Here's how the part is built. I have some questions about the finished solid (model axes, mm). A direction names the side the tool comes from. Give positions to 0.01 mm unless a question says otherwise; leave off trailing zeros. Loops run counter-clockwise (first coordinate to the right, second up) from the corner with the lowest first, then second, coordinate; pieces in that order, holes last.
Q1. I'm going to push flat-ended pins straight in: P1, Ø7.5, axis at x = -4.5, z = -5, coming from the +Y side; P2, Ø4, axis at x = 7.5, y = -52.5, coming from the +Z side (3 decimals); P3, Ø1, axis at x = 1.5, z = 5, coming from the +Y side. Where does each tip first touch, or does it pass through?
Q2. Suppose I cut it at A-A (z = 0). List the corners of the cut face in (x, y) for me, and give its area (3 significant figures).
Q3. Suppose I cut it at C-C (y = -17). List the corners of the cut face in (x, z) for me, and give its area (3 significant figures).
Q4. Thinking about a two-plate mould opening in Y: for faces 1 (the face through (0, -60, 0)), 2 (the face through (-2, 8, 0)), 3 (the face through (0, 12.3, 0)), which applies, pulls with the +Y half, pulls with the -Y half, needs draft (parallel to the pull), parting line crosses it, or undercut?
Q5. For faces 4 (the face through (3.755, -29.58, 11.923)), 5 (the face through (-3.417, 1.479, -0.759)), which set-ups out of +Z, -Z, +X, -X, +Y, -Y let a thin tool reach every point of the face, with its end or its side?
Q6. I need wall thicknesses on probe 1 along Y at (x, z) = (5.5, -2); probe 2 along X at (y, z) = (-38, 0); probe 3 along Z at (x, y) = (9, -40). Which ranges of each line are inside material? Lowest first, please.
Q7. Suppose I cut it at D-D (z = -7.5). List the corners of the cut face in (x, y) for me.
Q8. Suppose I cut it at B-B (x = 0). List the corners of the cut face in (y, z) for me.
```python
from build123d import *

# Parameters (mm, degrees)
SKETCH1_R           = 12.5
BOSS_EXTRUDE1_DEPTH = 60
SKETCH2_R           = 3.5
BOSS_EXTRUDE2_DEPTH = 3
SKETCH3_R           = 2
BOSS_EXTRUDE3_DEPTH = 9.3


with BuildPart() as part:
    # Sketch1 → Boss-Extrude1 (new body)
    with BuildSketch(Plane(origin=(0, 0, 0), x_dir=(1, 0, 0), z_dir=(0, 1, 0))):
        with Locations(Location((0, 0, 0), (0, 0, 270))):
            Circle(SKETCH1_R)
    extrude(amount=-BOSS_EXTRUDE1_DEPTH)

    # Sketch2 → Boss-Extrude2 (add)
    with BuildSketch(Plane(origin=(0, 0, 0), x_dir=(1, 0, 0), z_dir=(0, 1, 0))):
        with Locations(Location((0, 0, 0), (0, 0, 270))):
            Circle(SKETCH2_R)
    extrude(amount=BOSS_EXTRUDE2_DEPTH)

    # Sketch3 → Boss-Extrude3 (add)
    with BuildSketch(Plane(origin=(0, 3, 0), x_dir=(1, 0, 0), z_dir=(0, 1, 0))):
        with Locations(Location((0, 0, 0), (0, 0, 270))):
            Circle(SKETCH3_R)
    extrude(amount=BOSS_EXTRUDE3_DEPTH)


solid = part.part
```
Solutions:
1. P1: stops at y = 3
1. P2: stops at z = 11.225
1. P3: stops at y = 0
2. outline: (-12.5, -60) - (12.5, -60) - (12.5, 0) - (3.5, 0) - (3.5, 3) - (2, 3) - (2, 12.3) - (-2, 12.3) - (-2, 3) - (-3.5, 3) - (-3.5, 0) - (-12.5, 0) - close
2. area: 1,560 mm2
3. outline: circle Ø25 at (0, 0)
3. area: 491 mm2
4. face 1: pulls with the -Y half
4. face 2: needs draft
4. face 3: pulls with the +Y half
5. face 4: +Y, -Y
5. face 5: +Y
6. probe 1: y = -60 to 0
6. probe 2: x = -12.5 to 12.5
6. probe 3: z = -8.67 to 8.67
7. outline: (-10, -60) - (10, -60) - (10, 0) - (-10, 0) - close
8. outline: (-60, -12.5) - (0, -12.5) - (0, -3.5) - (3, -3.5) - (3, -2) - (12.3, -2) - (12.3, 2) - (3, 2) - (3, 3.5) - (0, 3.5) - (0, 12.5) - (-60, 12.5) - close
